Verification items for the finished model (mm, model axes). Face numbers are marked on the shaded views. A direction names the side the tool comes from. Give positions to 0.01 mm unless a question says otherwise; leave off trailing zeros. Return JSON: item names as keys, results as strings. Group by question number.
(1) Depth check by flat-ended pin: pin 1 Ø2 at (x, z) = (-3, 5) entering from +Y; pin 2 Ø6 at (x, z) = (1.5, 2.5) entering from +Y; pin 3 Ø3.5 at (x, z) = (-0.5, 7) entering from -Y; pin 4 Ø15.5 at (x, y) = (1.5, -6) entering from -Z. Enter the tip coordinate at first touch or a pass-through.
(2) Tool access check on the marked faces 1, 2 and 3. Record the directions out of +Z, -Z, +X, -X, +Y, -Y that give a thin tool (end or side, any length) a straight path to the whole face; none if there is none.
(3) Thickness scan on line 1 along Z through (x, y) = (12, 3); line 2 along Y through (x, z) = (2, 2.75); line 3 along Y through (x, z) = (0, 9). Record the ranges inside material, lowest first.
(4) Release check for a two-part mould opening along X. For the marked faces 4 and 5 record: pulls with the +X half, pulls with the -X half, needs draft (parallel to the pull), parting line crosses it, or undercut.
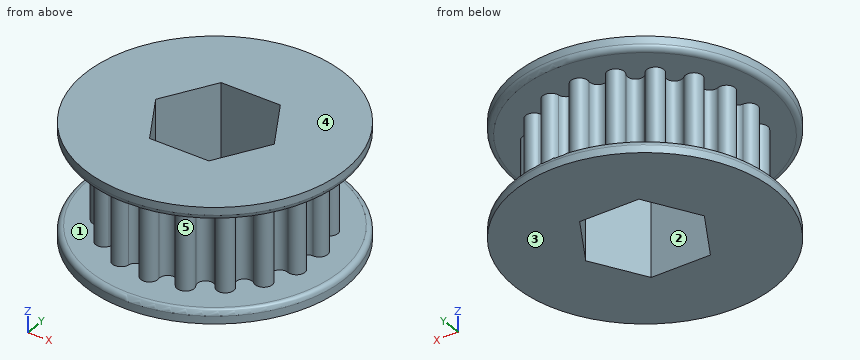
from build123d import *

# Parameters (mm, degrees)
BOSS_EXTRUDE1_DEPTH  = 10.922
SKETCH2_R            = 16.002
BOSS_EXTRUDE2_DEPTH  = 1.5875
FILLET1_R            = 0.635
FILLET1_OF_MIRROR1_R = 0.635


with BuildPart() as part:
    # Sketch1 → Boss-Extrude1 (new body)
    with BuildSketch(Plane.XY):
        with BuildLine():
            ThreePointArc((1.023014865, 11.438350063), (0, 12.7), (-1.023014865, 11.438350063))
            ThreePointArc((-1.023014865, 11.438350063), (-1.811146799, 10.271523911), (-2.950826609, 11.098424839))
            ThreePointArc((-2.950826609, 11.098424839), (-4.34365582, 11.934096284), (-4.873465647, 10.398641458))
            ThreePointArc((-4.873465647, 10.398641458), (-5.214989362, 9.032626536), (-6.568754843, 9.419865784))
            ThreePointArc((-6.568754843, 9.419865784), (-8.163402643, 9.728764428), (-8.136104548, 8.104703225))
            ThreePointArc((-8.136104548, 8.104703225), (-7.989827243, 6.704261093), (-9.3943943, 6.605131893))
            ThreePointArc((-9.3943943, 6.605131893), (-10.998522628, 6.35), (-10.417409164, 4.83321817))
            ThreePointArc((-10.417409164, 4.83321817), (-9.800974042, 3.567262818), (-11.086931157, 2.993721614))
            ThreePointArc((-11.086931157, 2.993721614), (-12.507058463, 2.205331856), (-11.442220491, 0.978775674))
            ThreePointArc((-11.442220491, 0.978775674), (-10.429978724, 0), (-11.442220491, -0.978775674))
            ThreePointArc((-11.442220491, -0.978775674), (-12.507058463, -2.205331856), (-11.086931157, -2.993721614))
            ThreePointArc((-11.086931157, -2.993721614), (-9.800974042, -3.567262818), (-10.417409164, -4.83321817))
            ThreePointArc((-10.417409164, -4.83321817), (-10.998522628, -6.35), (-9.3943943, -6.605131893))
            ThreePointArc((-9.3943943, -6.605131893), (-7.989827243, -6.704261093), (-8.136104548, -8.104703225))
            ThreePointArc((-8.136104548, -8.104703225), (-8.163402643, -9.728764428), (-6.568754843, -9.419865784))
            ThreePointArc((-6.568754843, -9.419865784), (-5.214989362, -9.032626536), (-4.873465647, -10.398641458))
            ThreePointArc((-4.873465647, -10.398641458), (-4.34365582, -11.934096284), (-2.950826609, -11.098424839))
            ThreePointArc((-2.950826609, -11.098424839), (-1.811146799, -10.271523911), (-1.023014865, -11.438350063))
            ThreePointArc((-1.023014865, -11.438350063), (0, -12.7), (1.023014865, -11.438350063))
            ThreePointArc((1.023014865, -11.438350063), (1.811146799, -10.271523911), (2.950826609, -11.098424839))
            ThreePointArc((2.950826609, -11.098424839), (4.34365582, -11.934096284), (4.873465647, -10.398641458))
            ThreePointArc((4.873465647, -10.398641458), (5.214989362, -9.032626536), (6.568754843, -9.419865784))
            ThreePointArc((6.568754843, -9.419865784), (8.163402643, -9.728764428), (8.136104548, -8.104703225))
            ThreePointArc((8.136104548, -8.104703225), (7.989827243, -6.704261093), (9.3943943, -6.605131893))
            ThreePointArc((9.3943943, -6.605131893), (10.998522628, -6.35), (10.417409164, -4.83321817))
            ThreePointArc((10.417409164, -4.83321817), (9.800974042, -3.567262818), (11.086931157, -2.993721614))
            ThreePointArc((11.086931157, -2.993721614), (12.507058463, -2.205331856), (11.442220491, -0.978775674))
            ThreePointArc((11.442220491, -0.978775674), (10.429978724, 0), (11.442220491, 0.978775674))
            ThreePointArc((11.442220491, 0.978775674), (12.507058463, 2.205331856), (11.086931157, 2.993721614))
            ThreePointArc((11.086931157, 2.993721614), (9.800974042, 3.567262818), (10.417409164, 4.83321817))
            ThreePointArc((10.417409164, 4.83321817), (10.998522628, 6.35), (9.3943943, 6.605131893))
            ThreePointArc((9.3943943, 6.605131893), (7.989827243, 6.704261093), (8.136104548, 8.104703225))
            ThreePointArc((8.136104548, 8.104703225), (8.163402643, 9.728764428), (6.568754843, 9.419865784))
            ThreePointArc((6.568754843, 9.419865784), (5.214989362, 9.032626536), (4.873465647, 10.398641458))
            ThreePointArc((4.873465647, 10.398641458), (4.34365582, 11.934096284), (2.950826609, 11.098424839))
            ThreePointArc((2.950826609, 11.098424839), (1.811146799, 10.271523911), (1.023014865, 11.438350063))
        make_face()
        Polygon((7.332348419, 0), (3.666174209, 6.35), (-3.666174209, 6.35), (-7.332348419, 0), (-3.666174209, -6.35), (3.666174209, -6.35), align=None, mode=Mode.SUBTRACT)
    extrude(amount=BOSS_EXTRUDE1_DEPTH)

    # Sketch2 → Boss-Extrude2 (add)
    with BuildSketch(Plane.XY.offset(10.922)):
        Circle(SKETCH2_R)
        Polygon((-3.666174209, 6.35), (-7.332348419, 0), (-3.666174209, -6.35), (3.666174209, -6.35), (7.332348419, 0), (3.666174209, 6.35), align=None, mode=Mode.SUBTRACT)
    boss_extrude2 = extrude(amount=BOSS_EXTRUDE2_DEPTH)

    # Fillet1
    fillet1_edges = [part.edges().sort_by_distance(p)[0] for p in [
        (-16.002, 0, 10.922),
    ]]
    fillet(fillet1_edges, radius=FILLET1_R)

    # Mirror1: Boss-Extrude2 across plane
    add(boss_extrude2.mirror(Plane.XY.offset(5.461)))

    # Fillet1 of Mirror1
    fillet1_of_mirror1_edges = [part.edges().sort_by_distance(p)[0] for p in [
        (-16.002, 0, 0),
    ]]
    fillet(fillet1_of_mirror1_edges, radius=FILLET1_OF_MIRROR1_R)


solid = part.part
Verdict:
{
 "1": {"pin 1": "y = 12", "pin 2": "y = 15.95", "pin 3": "y = -12.7", "pin 4": "z = -1.59"},
 "2": {"face 1": "none", "face 2": "+Z, -Z", "face 3": "-Z, +X, -X, +Y, -Y"},
 "3": {"line 1": "-1.59 to 0, 10.92 to 12.51", "line 2": "-10.26 to -6.35, 6.35 to 10.26", "line 3": "-12.7 to -6.35, 6.35 to 12.7"},
 "4": {"face 4": "needs draft", "face 5": "undercut"}
}
